Geometry: final body of the model. Coordinates: model frame, mm. Give positions to 0.01 mm unless a question says otherwise; leave off trailing zeros. Loops run counter-clockwise (first coordinate to the right, second up) from the corner with the lowest first, then second, coordinate; pieces in that order, holes last. Notation, with made-up numbers: (69.25, 53) - (128.25, 53) arc R31 ccw to (128.25, 77) - close; hole circle Ø2 at (55, 12). An arc over 180 degrees is marked (long way). Answer in a Markdown table with one row per item.
from build123d import *

# Parameters (mm, degrees)
SKETCH_1_W      = 110
SKETCH_1_H      = 70
SKETCH_1_R      = 1.55
EXTRUDE_1_DEPTH = 0.8
FILLET_1_R      = 2
FILLET_2_R      = 2
FILLET_3_R      = 2
FILLET_4_R      = 2


with BuildPart() as part:
    # 草图1 → 凸台-拉伸1 (new body)
    with BuildSketch(Plane(origin=(0, 0, 0), x_dir=(1, 0, 0), z_dir=(0, 1, 0))):
        Rectangle(SKETCH_1_W, SKETCH_1_H)
        with Locations(Location((-49, 30, 0), (0, 0, 270))):
            Circle(SKETCH_1_R, mode=Mode.SUBTRACT)
        with Locations(Location((49, 30, 0), (0, 0, 90))):
            Circle(SKETCH_1_R, mode=Mode.SUBTRACT)
        with Locations(Location((49, -30, 0), (0, 0, 270))):
            Circle(SKETCH_1_R, mode=Mode.SUBTRACT)
        with Locations(Location((-49, -30, 0), (0, 0, 90))):
            Circle(SKETCH_1_R, mode=Mode.SUBTRACT)
        with Locations(Location((-42.5, 25.5, 0), (0, 0, 270))):
            Circle(SKETCH_1_R, mode=Mode.SUBTRACT)
        with Locations(Location((42.5, 25.5, 0), (0, 0, 90))):
            Circle(SKETCH_1_R, mode=Mode.SUBTRACT)
        with Locations(Location((42.5, -25.5, 0), (0, 0, 270))):
            Circle(SKETCH_1_R, mode=Mode.SUBTRACT)
        with Locations(Location((-42.5, -25.5, 0), (0, 0, 90))):
            Circle(SKETCH_1_R, mode=Mode.SUBTRACT)
        with BuildLine():
            Line((-7, 30.023350274), (7, 30.023350274))
            ThreePointArc((7, 30.023350274), (8.55, 28.473350274), (7, 26.923350274))
            Line((7, 26.923350274), (-7, 26.923350274))
            ThreePointArc((-7, 26.923350274), (-8.55, 28.473350274), (-7, 30.023350274))
        make_face(mode=Mode.SUBTRACT)
        with BuildLine():
            Line((7, -26.923350274), (-7, -26.923350274))
            ThreePointArc((-7, -26.923350274), (-8.55, -28.473350274), (-7, -30.023350274))
            Line((-7, -30.023350274), (7, -30.023350274))
            ThreePointArc((7, -30.023350274), (8.55, -28.473350274), (7, -26.923350274))
        make_face(mode=Mode.SUBTRACT)
    extrude(amount=EXTRUDE_1_DEPTH)

    # 圆角1
    fillet_1_edges = [part.edges().sort_by_distance(p)[0] for p in [
        (55, 0.4, -35),
    ]]
    fillet(fillet_1_edges, radius=FILLET_1_R)

    # 圆角2
    fillet_2_edges = [part.edges().sort_by_distance(p)[0] for p in [
        (-55, 0.4, -35),
    ]]
    fillet(fillet_2_edges, radius=FILLET_2_R)

    # 圆角3
    fillet_3_edges = [part.edges().sort_by_distance(p)[0] for p in [
        (-55, 0.4, 35),
    ]]
    fillet(fillet_3_edges, radius=FILLET_3_R)

    # 圆角4
    fillet_4_edges = [part.edges().sort_by_distance(p)[0] for p in [
        (55, 0.4, 35),
    ]]
    fillet(fillet_4_edges, radius=FILLET_4_R)


solid = part.part
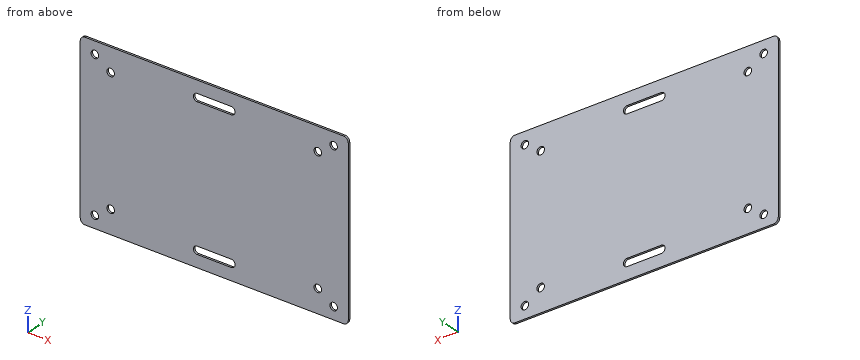
Q1. Cut plane C-C (z = 25.5). Output: boundary loops of the cut face in (x, y), and give its area (3 significant figures).
Check values:
| item | result |
|---|---|
| outline | (-55, 0) - (-44.05, 0) - (-44.05, 0.8) - (-55, 0.8) - close; (-40.95, 0) - (40.95, 0) - (40.95, 0.8) - (-40.95, 0.8) - close; (44.05, 0) - (55, 0) - (55, 0.8) - (44.05, 0.8) - close |
| area | 83.0 mm² |
Q2. Cut plane A-A (y = 0.25). Give the number of separate pieces and of enclosed holes in the cut face, and give its area (3 significant figures).
Check values:
| item | result |
|---|---|
| separate pieces | 1 |
| enclosed holes | 10 |
| area | 7,530 mm² |
Q3. Cut plane B-B (x = -2.5). Output: boundary loops of the cut face in (y, z).
Check values:
| item | result |
|---|---|
| outline | (0, -35) - (0.8, -35) - (0.8, -30.02) - (0, -30.02) - close; (0, -26.92) - (0.8, -26.92) - (0.8, 26.92) - (0, 26.92) - close; (0, 30.02) - (0.8, 30.02) - (0.8, 35) - (0, 35) - close |
Q4. Material intervals for line 1 along Z through (x, y) = (-1, 0.4); line 2 along X through (y, z) = (0.55, 25.5), sorted ascending.
Check values:
| item | result |
|---|---|
| line 1 | -35 to -30.02, -26.92 to 26.92, 30.02 to 35 |
| line 2 | -55 to -44.05, -40.95 to 40.95, 44.05 to 55 |
